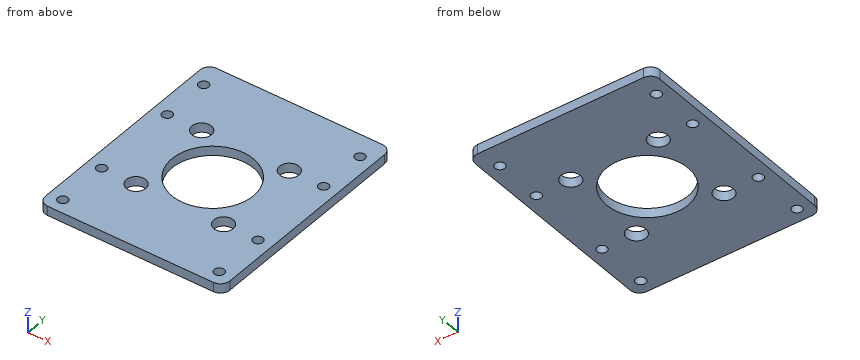
Autodesk Inventor part; units mm, degrees
ref_plane "YZ Plane" through (0, 0, 0) normal (1, 0, 0) x (0, 1, 0)
ref_plane "XZ Plane" through (0, 0, 0) normal (0, 1, 0) x (-1, 0, 0)
ref_plane "XY Plane" through (0, 0, 0) normal (0, 0, 1) x (1, 0, 0)
sketch "スケッチ1" plane through (0, 0, 0) normal (0, 0, 1) x (1, 0, 0)
  circle A0 centre (0, 0) radius 13
  circle A1 centre (-14, 14) radius 3.1
  circle A2 centre (14, 14) radius 3.1
  circle A3 centre (-14, -14) radius 3.1
  circle A4 centre (14, -14) radius 3.1
  line L0 (20, 20) -> (-20, 20) construction
  line L1 (-20, 20) -> (-20, -20) construction
  line L2 (-20, -20) -> (20, -20) construction
  line L3 (20, -20) -> (20, 20) construction
  line L4 (20, 20) -> (-20, -20) construction
  line L5 (-20, 20) -> (20, -20) construction
  circle A5 centre (-25, 14) radius 1.6
  circle A6 centre (-25, -14) radius 1.6
  circle A7 centre (25, 14) radius 1.6
  circle A8 centre (25, -14) radius 1.6
  line L6 (-47.387, 37) -> (51.5127, 37) construction
  line L7 (51.5127, 37) -> (51.5127, 22) construction
  line L8 (51.5127, 22) -> (-47.387, 22) construction
  line L9 (-47.387, 22) -> (-47.387, 37) construction
  circle A9 centre (-25, 29.5) radius 1.6
  circle A10 centre (25, 29.5) radius 1.6
  circle A11 centre (-25, -30.5) radius 1.6
  circle A12 centre (25, -30.5) radius 1.6
  line L10 (-36.8919, -26) -> (36.9631, -26) construction
  line L11 (36.9631, -26) -> (36.9631, -35) construction
  line L12 (36.9631, -35) -> (-36.8919, -35) construction
  line L13 (-36.8919, -35) -> (-36.8919, -26) construction
  line L14 (-29.5, 37) -> (-29.5, -35)
  line L15 (-29.5, 37) -> (29.5, 37)
  line L16 (29.5, 37) -> (29.5, -35)
  line L17 (-29.5, -35) -> (29.5, -35)
  dimension "d0" = 26
  dimension "d1" = 6.2
  dimension "d2" = 6.2
  dimension "d3" = 6.2
  dimension "d4" = 6.2
  dimension "d5" = 28
  dimension "d6" = 28
  dimension "d7" = 14
  dimension "d8" = 14
  dimension "d9" = 40
  dimension "d10" = 40
  dimension "d11" = 3.2
  dimension "d12" = 3.2
  dimension "d13" = 3.2
  dimension "d14" = 3.2
  dimension "d15" = 15
  dimension "d16" = 2
  dimension "d17" = 5
  dimension "d18" = 5
  dimension "d19" = 3.2
  dimension "d20" = 3.2
  dimension "d21" = 7.5
  dimension "d22" = 3.2
  dimension "d23" = 3.2
  dimension "d26" = 9
  dimension "d27" = 4.5
  dimension "d28" = 63
  dimension "d29" = 4.5
  dimension "d30" = 4.5
extrude "押し出し1" add sketch "スケッチ1" along normal blind 3
fillet "フィレット1" radius 3 4 edges at (-29.5, 37, 1.5) (29.5, 37, 1.5) (29.5, -35, 1.5) (-29.5, -35, 1.5)
properties part number "ハンド_シリンダ固定板" material "アルミニウム 6061"
Geometry: final body of the model. Coordinates: model frame, mm. Round coordinates to 2 decimals unless told otherwise and drop trailing zeros. Loops run counter-clockwise (first coordinate to the right, second up) from the corner with the lowest first, then second, coordinate; pieces in that order, holes last.
Q1. Section D-D on x = 25. Return loops of the section in (y, z).
Q2. Section C-C on y = 0. Return loops of the section in (x, z), plus the area to 3 significant figures.
Q3. Section B-B on x = 0. Return loops of the section in (y, z).
Q4. Material intervals for L1, parallel to Y at x = -4.5, z = 1.8; L2, parallel to Y at x = -3, z = 0.2, sorted ascending.
Q5. Section A-A on y = 29.5. Return loops of the section in (x, z).
Evaluation:
1. outline: (-35, 0) - (-32.1, 0) - (-32.1, 3) - (-35, 3) - close; (-28.9, 0) - (-15.6, 0) - (-15.6, 3) - (-28.9, 3) - close; (-12.4, 0) - (12.4, 0) - (12.4, 3) - (-12.4, 3) - close; (15.6, 0) - (27.9, 0) - (27.9, 3) - (15.6, 3) - close; (31.1, 0) - (37, 0) - (37, 3) - (31.1, 3) - close
2. outline: (-29.5, 0) - (-13, 0) - (-13, 3) - (-29.5, 3) - close; (13, 0) - (29.5, 0) - (29.5, 3) - (13, 3) - close
2. area: 99.0 mm2
3. outline: (-35, 0) - (-13, 0) - (-13, 3) - (-35, 3) - close; (13, 0) - (37, 0) - (37, 3) - (13, 3) - close
4. L1: y = -35 to -12.2, 12.2 to 37
4. L2: y = -35 to -12.65, 12.65 to 37
5. outline: (-29.5, 0) - (-26.6, 0) - (-26.6, 3) - (-29.5, 3) - close; (-23.4, 0) - (23.4, 0) - (23.4, 3) - (-23.4, 3) - close; (26.6, 0) - (29.5, 0) - (29.5, 3) - (26.6, 3) - close
